Part model, mm, in its own coordinate system. A direction names the side the tool comes from. Coordinates: 2 decimals unless noted, no trailing zeros. Loops run counter-clockwise (first coordinate to the right, second up) from the corner with the lowest first, then second, coordinate; pieces in that order, holes last. Notation, with made-up numbers: M -28,69 L 6,69 A17 ccw 6,73 Z; hole C -8,-11 d4. An arc over 180 degrees is marked long. Use a Markdown table: item, result. Add a question column.
1) Wall check: probe 1 along Y at (x, z) = (0, -10.95); probe 2 along Z at (x, y) = (-10, 31.5); probe 3 along X at (y, z) = (13.75, 0). Give the ranges that are in metal, low to high. Write a range as from..to.
2) Band-saw the part on C-C (z = 1). List the corners of the cut face in (x, y), plus the area to 3 significant figures.
3) Pin check, flat tips, straight feed: pin 1 Ø1.5 at (x, z) = (3, -1.5) entering from +Y; pin 2 Ø4.5 at (x, y) = (0, 30) entering from +Z; pin 3 Ø8 at (x, z) = (3, 4.5) entering from +Y. Stop position of each tip, or through.
4) Band-saw the part on A-A (y = 22.5). List the corners of the cut face in (x, z), plus the area to 3 significant figures.
5) Band-saw the part on B-B (x = 0). List the corners of the cut face in (y, z).
6) Pull direction X, two halves, no side cores. Call faces 1 (the cylindrical face through (0, 41, 10)), 2 (the flat face through (0, 21, -12)), 3 (the cylindrical face through (-3.905, 8.619, -0.867)): released by +X, released by -X, zero draft, split by the parting line, or undercut.
7) Band-saw the part on D-D (y = 4). List the corners of the cut face in (x, z), plus the area to 3 significant figures.
8) Tool access for faces 4 (the cylindrical face through (0, 41, -10)), 5 (the flat face through (0, 26, 8)): list every direction of +Z, -Z, +X, -X, +Y, -Y with a clear straight run to the whole face (end or side of a thin tool).
from build123d import *

# Parameters (mm, degrees)
CROQUIS1_W              = 22
CROQUIS1_H              = 24
SALIENTE_EXTRUIR1_DEPTH = 30
SALIENTE_EXTRUIR2_DEPTH = 24
CROQUIS4_W              = 16
CROQUIS4_H              = 27.551854113
CORTAR_EXTRUIR1_DEPTH   = 24
CROQUIS5_R              = 4
CORTAR_EXTRUIR2_DEPTH   = 24
CROQUIS6_R              = 2.5
CORTAR_EXTRUIR3_DEPTH   = 49.764741361


with BuildPart() as part:
    # Croquis1 → Saliente-Extruir1 (new body)
    with BuildSketch(Plane(origin=(0, 0, 0), x_dir=(1, 0, 0), z_dir=(0, 1, 0))):
        Rectangle(CROQUIS1_W, CROQUIS1_H)
    extrude(amount=SALIENTE_EXTRUIR1_DEPTH)

    # Croquis3 → Saliente-Extruir2 (add)
    with BuildSketch(Plane.XY.offset(12)):
        with BuildLine():
            Line((-11, 30), (11, 30))
            ThreePointArc((11, 30), (0, 41), (-11, 30))
        make_face()
    extrude(amount=-SALIENTE_EXTRUIR2_DEPTH)

    # Croquis4 → Cortar-Extruir1 (cut)
    with BuildSketch(Plane(origin=(11, 0, 0), x_dir=(0, 0, -1), z_dir=(1, 0, 0))):
        with Locations((0, 30.775927057)):
            Rectangle(CROQUIS4_W, CROQUIS4_H)
    extrude(amount=-CORTAR_EXTRUIR1_DEPTH, mode=Mode.SUBTRACT)

    # Croquis5 → Cortar-Extruir2 (cut)
    with BuildSketch(Plane(origin=(0, 17, 0), x_dir=(1, 0, 0), z_dir=(0, 1, 0))):
        with Locations(Location((0, 0, 0), (0, 0, 270))):
            Circle(CROQUIS5_R)
    extrude(amount=-CORTAR_EXTRUIR2_DEPTH, mode=Mode.SUBTRACT)

    # Croquis6 → Cortar-Extruir3 (cut, through all)
    with BuildSketch(Plane.XY.offset(12)):
        with Locations((0, 30)):
            Circle(CROQUIS6_R)
    extrude(amount=-CORTAR_EXTRUIR3_DEPTH, mode=Mode.SUBTRACT)


solid = part.part
Entries:
| question | item | result |
|---|---|---|
| 1 | probe 1 | 0..27.5, 32.5..41 |
| 1 | probe 2 | -12..-8, 8..12 |
| 1 | probe 3 | -11..-4, 4..11 |
| 2 | outline | M -11,0 L -3.87,0 L -3.87,17 L -11,17 Z; M 3.87,0 L 11,0 L 11,17 L 3.87,17 Z |
| 2 | area | 242 mm2 |
| 3 | pin 1 | y = 17 |
| 3 | pin 2 | through |
| 3 | pin 3 | y = 40.95 |
| 4 | outline | M -11,-12 L 11,-12 L 11,-8 L -11,-8 Z; M -11,8 L 11,8 L 11,12 L -11,12 Z |
| 4 | area | 176 mm2 |
| 5 | outline | M 0,-12 L 27.5,-12 L 27.5,-8 L 17,-8 L 17,-4 L 0,-4 Z; M 0,4 L 17,4 L 17,8 L 27.5,8 L 27.5,12 L 0,12 Z; M 32.5,-12 L 41,-12 L 41,-8 L 32.5,-8 Z; M 32.5,8 L 41,8 L 41,12 L 32.5,12 Z |
| 6 | face 1 | split by the parting line |
| 6 | face 2 | zero draft |
| 6 | face 3 | undercut |
| 7 | outline | M -11,-12 L 11,-12 L 11,12 L -11,12 Z; hole C 0,0 d8 |
| 7 | area | 478 mm2 |
| 8 | face 4 | +Z, -Z, +Y |
| 8 | face 5 | +X, -X, +Y |
